from build123d import *

# Parameters (mm, degrees)
SKETCH4_R           = 0.9
BOSS_EXTRUDE1_DEPTH = 1


with BuildPart() as part:
    # Sketch1 → Revolve1 (revolve)
    with BuildSketch(Plane.XY):
        with BuildLine():
            Line((0, 29.75), (13, 29.75))
            Line((13, 29.75), (13, 30))
            Line((13, 30), (14.3, 30))
            ThreePointArc((14.3, 30), (14.794974747, 29.794974747), (15, 29.3))
            Line((15, 29.3), (15, 5.390363203))
            ThreePointArc((15, 5.390363203), (14.990192231, 5.321025678), (14.961538462, 5.257128525))
            ThreePointArc((14.961538462, 5.257128525), (14.5, 3.658312395), (14.961538462, 2.059496265))
            ThreePointArc((14.961538462, 2.059496265), (14.990192231, 1.995599112), (15, 1.926261588))
            Line((15, 1.926261588), (15, 0.25))
            ThreePointArc((15, 0.25), (14.926776695, 0.073223305), (14.75, 0))
            Line((14.75, 0), (0, 0))
            Line((0, 0), (0, 29.75))
        make_face()
    revolve(axis=Axis((0, 0, 0), (0, 1, 0)))

    # Sketch4 → Boss-Extrude1 (add)
    with BuildSketch(Plane.XZ):
        with Locations((5, 0)):
            Circle(SKETCH4_R)
        with Locations((-5, 0)):
            Circle(SKETCH4_R)
    extrude(amount=BOSS_EXTRUDE1_DEPTH)


solid = part.part
Model file for the job. Use its own axes, mm. A direction names the side the tool comes from. Round coordinates to 2 decimals unless told otherwise and drop trailing zeros. Order: outer loops, then holes, each group sorted by start corner. A loop starts at its lowest first (then second) coordinate and runs counter-clockwise, first axis right, second up.
(1) Pin check, flat tips, straight feed: pin 1 (1.5 mm diameter, centred on x = 8.5, z = -1.5, fed in from -Y); pin 2 (10 mm diameter, centred on y = 13.5, z = -10, fed in from -X); pin 3 (1.5 mm diameter, centred on y = 16.5, z = -7, fed in from -X); pin 4 (5 mm diameter, centred on x = -6, z = 1, fed in from -Y). Stop position of each tip, or through.
(2) Band-saw the part on C-C (y = 19). List the corners of the cut face in (x, z).
(3) Pull direction Z, two halves, no side cores. Call faces 1 (the face through (-14.985, 17.178, -0.66)), 2 (the face through (5, -1, 0)), 3 (the face through (0, 29.75, 0)): released by +Z, released by -Z, zero draft, split by the parting line, or undercut.
(4) Band-saw the part on A-A (z = 0). List the corners of the cut face in (x, y).
(5) Drill centre lines: line 1 (Y direction, x = -3.5, z = -8); line 2 (Z direction, x = 0, y = 29); line 3 (Y direction, x = 8.5, z = -10). Where is each one in solid material? Low to high.
(6) Band-saw the part on B-B (x = 0). List the corners of the cut face in (y, z).
(7) 3-axis set-ups, long thin cutter, end or side, ignore diameter. For faces 4 (the face through (-5.9, -0.5, 0)), 5 (the face through (-14.985, 1.076, -0.66)): which of +Z, -Z, +X, -X, +Y, -Y reach the whole face in a straight line?
Verdict:
1. pin 1: stops at y = 0
1. pin 2: stops at x = -14.14
1. pin 3: stops at x = -13.64
1. pin 4: stops at y = -1
2. outline: circle Ø30 at (0, 0)
3. face 1: split by the parting line
3. face 2: zero draft
3. face 3: undercut
4. outline: (-15, 0.25) arc R0.25 ccw to (-14.75, 0) - (-5.9, 0) - (-5.9, -1) - (-4.1, -1) - (-4.1, 0) - (4.1, 0) - (4.1, -1) - (5.9, -1) - (5.9, 0) - (14.75, 0) arc R0.25 ccw to (15, 0.25) - (15, 1.93) arc R0.25 ccw to (14.96, 2.06) arc R3 cw to (14.96, 5.26) arc R0.25 ccw to (15, 5.39) - (15, 29.3) arc R0.7 ccw to (14.3, 30) - (13, 30) - (13, 29.75) - (-13, 29.75) - (-13, 30) - (-14.3, 30) arc R0.7 ccw to (-15, 29.3) - (-15, 5.39) arc R0.25 ccw to (-14.96, 5.26) arc R3 cw to (-14.96, 2.06) arc R0.25 ccw to (-15, 1.93) - close
5. line 1: y = 0 to 29.75
5. line 2: z = -15 to 15
5. line 3: y = 0 to 30
6. outline: (0, -14.75) arc R0.25 ccw to (0.25, -15) - (1.93, -15) arc R0.25 ccw to (2.06, -14.96) arc R3 cw to (5.26, -14.96) arc R0.25 ccw to (5.39, -15) - (29.3, -15) arc R0.7 ccw to (30, -14.3) - (30, -13) - (29.75, -13) - (29.75, 13) - (30, 13) - (30, 14.3) arc R0.7 ccw to (29.3, 15) - (5.39, 15) arc R0.25 ccw to (5.26, 14.96) arc R3 cw to (2.06, 14.96) arc R0.25 ccw to (1.93, 15) - (0.25, 15) arc R0.25 ccw to (0, 14.75) - close
7. face 4: -Y
7. face 5: +Y, -Y
